from build123d import *

# Parameters (mm, degrees)
BOSS_EXTRUDE1_DEPTH = 2.8
BOSS_EXTRUDE2_DEPTH = 1
SKETCH3_W           = 32.16332029
SKETCH3_H           = 5.710000001
BOSS_EXTRUDE3_DEPTH = 5.8
CUT_EXTRUDE1_DEPTH  = 10


with BuildPart() as part:
    # Sketch1 → Boss-Extrude1 (new body)
    with BuildSketch(Plane.XY):
        with BuildLine():
            Line((-53.39, 36.695), (53.39, 36.695))
            ThreePointArc((53.39, 36.695), (54.528441918, 36.223441918), (55, 35.085))
            Line((55, 35.085), (55, -35.085))
            ThreePointArc((55, -35.085), (54.528441918, -36.223441918), (53.39, -36.695))
            Line((53.39, -36.695), (-53.39, -36.695))
            ThreePointArc((-53.39, -36.695), (-54.528441918, -36.223441918), (-55, -35.085))
            Line((-55, -35.085), (-55, 35.085))
            ThreePointArc((-55, 35.085), (-54.528441918, 36.223441918), (-53.39, 36.695))
        make_face()
    extrude(amount=BOSS_EXTRUDE1_DEPTH)

    # Sketch2 → Boss-Extrude2 (add)
    with BuildSketch(Plane.XY.offset(2.8)):
        with BuildLine():
            Line((25.241660148, 33.374999999), (25.241660148, 30.984999999))
            Line((25.241660148, 30.984999999), (14.471660145, 30.984999999))
            ThreePointArc((14.471660145, 30.984999999), (14.943218227, 29.846558082), (16.081660145, 29.374999999))
            Line((16.081660145, 29.374999999), (25.241660148, 29.374999999))
            ThreePointArc((25.241660148, 29.374999999), (26.380102065, 29.846558082), (26.851660148, 30.984999999))
            Line((26.851660148, 30.984999999), (26.851660148, 33.374999999))
            Line((26.851660148, 33.374999999), (51.679999999, 33.374999999))
            Line((51.679999999, 33.374999999), (51.679999999, -33.374999999))
            Line((51.679999999, -33.374999999), (-51.679999999, -33.374999999))
            Line((-51.679999999, -33.374999999), (-51.679999999, 33.374999999))
            Line((-51.679999999, 33.374999999), (-26.851660148, 33.374999999))
            Line((-26.851660148, 33.374999999), (-26.851660148, 30.984999999))
            ThreePointArc((-26.851660148, 30.984999999), (-26.380102065, 29.846558082), (-25.241660148, 29.374999999))
            Line((-25.241660148, 29.374999999), (-16.081660145, 29.374999999))
            ThreePointArc((-16.081660145, 29.374999999), (-14.943218227, 29.846558082), (-14.471660145, 30.984999999))
            Line((-14.471660145, 30.984999999), (-25.241660148, 30.984999999))
            Line((-25.241660148, 30.984999999), (-25.241660148, 33.374999999))
            ThreePointArc((-25.241660148, 33.374999999), (-25.71321823, 34.513441917), (-26.851660148, 34.984999999))
            Line((-26.851660148, 34.984999999), (-51.679999999, 34.984999999))
            ThreePointArc((-51.679999999, 34.984999999), (-52.818441916, 34.513441917), (-53.289999999, 33.374999999))
            Line((-53.289999999, 33.374999999), (-53.289999999, -33.374999999))
            ThreePointArc((-53.289999999, -33.374999999), (-52.818441916, -34.513441917), (-51.679999999, -34.984999999))
            Line((-51.679999999, -34.984999999), (51.679999999, -34.984999999))
            ThreePointArc((51.679999999, -34.984999999), (52.818441916, -34.513441917), (53.289999999, -33.374999999))
            Line((53.289999999, -33.374999999), (53.289999999, 33.374999999))
            ThreePointArc((53.289999999, 33.374999999), (52.818441916, 34.513441917), (51.679999999, 34.984999999))
            Line((51.679999999, 34.984999999), (26.851660148, 34.984999999))
            ThreePointArc((26.851660148, 34.984999999), (25.71321823, 34.513441917), (25.241660148, 33.374999999))
        make_face()
    extrude(amount=BOSS_EXTRUDE2_DEPTH)

    # Sketch3 → Boss-Extrude3 (add)
    with BuildSketch(Plane.XY.offset(2.8)):
        with Locations((0, 33.84)):
            Rectangle(SKETCH3_W, SKETCH3_H)
    extrude(amount=BOSS_EXTRUDE3_DEPTH)

    # Sketch4 → Cut-Extrude1 (cut)
    with BuildSketch(Plane(origin=(0, 36.695, 0), x_dir=(1, 0, 0), z_dir=(0, 1, 0))):
        with BuildLine():
            Line((-16.081660145, -8.479373109), (-16.081660145, -8.6))
            Line((-16.081660145, -8.6), (16.081660145, -8.6))
            Line((16.081660145, -8.6), (16.081660145, -8.479373109))
            ThreePointArc((16.081660145, -8.479373109), (0, -2.41), (-16.081660145, -8.479373109))
        make_face()
    extrude(amount=-CUT_EXTRUDE1_DEPTH, mode=Mode.SUBTRACT)


solid = part.part
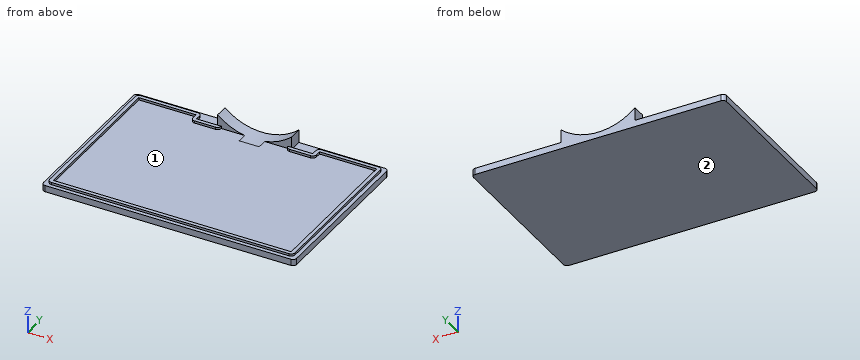
Work out the finished part from the listing and answer in its coordinate system (mm). Face numbers are marked on the shaded views. Give positions to 0.01 mm unless a question says otherwise; leave off trailing zeros. Loops run counter-clockwise (first coordinate to the right, second up) from the corner with the lowest first, then second, coordinate; pieces in that order, holes last. Notation, with made-up numbers: (60.5, 70) -> (70.5, 70) arc R6 cw to (70.5, 76) -> close; hole circle Ø11 at (-14, 59). An arc over 180 degrees is marked (long way). Use a Markdown table: item, result. Add a question column.
1) Consider line 1 along Z through (x, y) = (-49, -20); line 2 along Y through (x, z) = (12, 5.5) (3 decimals); line 3 along X through (y, z) = (19, 3.5). Determine where each line is inside the solid, lowest interval first.
2) The part is cut by section A-A, the plane z = 7. Determine the outline of the cut face in (x, y) (3 decimals), plus the area to 3 significant figures.
3) The part is cut by section B-B, the plane x = 39. Determine the outline of the cut face in (y, z) (3 decimals).
4) The part is cut by section D-D, the plane x = 11.5. Determine the outline of the cut face in (y, z) (3 decimals), plus the area to 3 significant figures.
5) The part is cut by section C-C, the plane y = 9. Determine the outline of the cut face in (x, z), plus the area to 3 significant figures.
6) Each of these flat-tipped pins is pushed along its axis until it touches: P1, Ø0.8, axis at y = 32, z = 3.5, coming from the +X side; P2, Ø1.5, axis at y = 2.5, z = 6, coming from the +X side; P3, Ø0.5, axis at x = -21, z = 3.5, coming from the -Y side (3 decimals); P4, Ø0.5, axis at y = 32.5, z = 3.5, coming from the -X side. Where does it stop, or does it pass through?
7) For a pull along Y with two mould halves and no side action, classify the marked faces 1 and 2 as +Y half, -Y half, draft (parallel to the pull), parting line (faces both ways), or undercut.
Reported:
| question | item | result |
|---|---|---|
| 1 | line 1 | z = 0 to 2.8 |
| 1 | line 2 | y = 30.985 to 36.695 |
| 1 | line 3 | x = -53.29 to -51.68, 51.68 to 53.29 |
| 2 | outline | (-16.082, 30.985) -> (-14.226, 30.985) -> (-14.226, 36.695) -> (-16.082, 36.695) -> close; (14.226, 30.985) -> (16.082, 30.985) -> (16.082, 36.695) -> (14.226, 36.695) -> close |
| 2 | area | 21.2 mm^2 |
| 3 | outline | (-36.695, 0) -> (36.695, 0) -> (36.695, 2.8) -> (34.985, 2.8) -> (34.985, 3.8) -> (33.375, 3.8) -> (33.375, 2.8) -> (-33.375, 2.8) -> (-33.375, 3.8) -> (-34.985, 3.8) -> (-34.985, 2.8) -> (-36.695, 2.8) -> close |
| 4 | outline | (-36.695, 0) -> (36.695, 0) -> (36.695, 5.298) -> (30.985, 5.298) -> (30.985, 2.8) -> (-33.375, 2.8) -> (-33.375, 3.8) -> (-34.985, 3.8) -> (-34.985, 2.8) -> (-36.695, 2.8) -> close |
| 4 | area | 221 mm^2 |
| 5 | outline | (-55, 0) -> (55, 0) -> (55, 2.8) -> (53.29, 2.8) -> (53.29, 3.8) -> (51.68, 3.8) -> (51.68, 2.8) -> (-51.68, 2.8) -> (-51.68, 3.8) -> (-53.29, 3.8) -> (-53.29, 2.8) -> (-55, 2.8) -> close |
| 5 | area | 311 mm^2 |
| 6 | P1 | stops at x = 53.29 |
| 6 | P2 | passes through |
| 6 | P3 | stops at y = -34.985 |
| 6 | P4 | stops at x = -53.29 |
| 7 | face 1 | undercut |
| 7 | face 2 | draft |
